Build history of the part. All positions in model axes, mm. Round coordinates to 2 decimals unless told otherwise and drop trailing zeros. Order: outer loops, then holes, each group sorted by start corner. A loop starts at its lowest first (then second) coordinate and runs counter-clockwise, first axis right, second up. Notation, with made-up numbers: (70.5, 13.5) -> (123.5, 13.5) arc R29 cw to (123.5, 43.5) -> close; hole circle Ø3 at (-18.75, -2). An arc over 180 degrees is marked (long way). Write item = value, one per line.
from build123d import *

# Parameters (mm, degrees)
SKETCH1_W           = 120
SKETCH1_H           = 120
BOSS_EXTRUDE1_DEPTH = 2
SKETCH2_R           = 1.775
CUT_EXTRUDE1_DEPTH  = 182.037166061
SKETCH3_R           = 1.775
CUT_EXTRUDE2_DEPTH  = 182.037166061
SKETCH4_W           = 3.55
SKETCH4_H           = 28
CUT_EXTRUDE3_DEPTH  = 182.037166061


with BuildPart() as part:
    # Sketch1 → Boss-Extrude1 (new body)
    with BuildSketch(Plane(origin=(0, 0, 0), x_dir=(1, 0, 0), z_dir=(0, 1, 0))):
        with Locations((104.879995502, 14.733142437)):
            Rectangle(SKETCH1_W, SKETCH1_H)
    extrude(amount=BOSS_EXTRUDE1_DEPTH)

    # Sketch2 → Cut-Extrude1 (cut, through all)
    with BuildSketch(Plane(origin=(0, 2, 0), x_dir=(1, 0, 0), z_dir=(0, 1, 0))):
        with Locations(Location((65.379995502, 30.733142437, 0), (0, 0, 270))):
            Circle(SKETCH2_R)
        with Locations(Location((65.379995502, -1.266857563, 0), (0, 0, 270))):
            Circle(SKETCH2_R)
        with Locations(Location((144.379995502, -1.266857563, 0), (0, 0, 270))):
            Circle(SKETCH2_R)
        with Locations(Location((144.379995502, 30.733142437, 0), (0, 0, 270))):
            Circle(SKETCH2_R)
    extrude(amount=-CUT_EXTRUDE1_DEPTH, mode=Mode.SUBTRACT)

    # Sketch3 → Cut-Extrude2 (cut, through all)
    with BuildSketch(Plane(origin=(0, 2, 0), x_dir=(1, 0, 0), z_dir=(0, 1, 0))):
        with Locations(Location((87.379995502, -24.766857563, 0), (0, 0, 270))):
            Circle(SKETCH3_R)
        with Locations(Location((87.379995502, 54.233142437, 0), (0, 0, 270))):
            Circle(SKETCH3_R)
        with Locations(Location((122.379995502, -24.766857563, 0), (0, 0, 270))):
            Circle(SKETCH3_R)
        with Locations(Location((122.379995502, 54.233142437, 0), (0, 0, 270))):
            Circle(SKETCH3_R)
    extrude(amount=-CUT_EXTRUDE2_DEPTH, mode=Mode.SUBTRACT)

    # Sketch4 → Cut-Extrude3 (cut, through all)
    with BuildSketch(Plane(origin=(0, 2, 0), x_dir=(1, 0, 0), z_dir=(0, 1, 0))):
        with Locations((78.879995502, 11.820412138)):
            Rectangle(SKETCH4_W, SKETCH4_H)
        with Locations((130.879995502, 11.820412138)):
            Rectangle(SKETCH4_W, SKETCH4_H)
    extrude(amount=-CUT_EXTRUDE3_DEPTH, mode=Mode.SUBTRACT)


solid = part.part
Q1. Mould opens along Z. For faces 1 (the face through (104, 0, -16)), 2 (the face through (146.14, 1.01, 1.04)), 3 (the face through (121.7, 1.014, 26.407)) say: released by +Z, released by -Z, zero draft, split by the parting line, or undercut.
Check values:
face_1 = zero draft
face_2 = undercut
face_3 = undercut
Q2. Flat gauge pin, fed straight in: pin 1 (2 mm diameter, centred on x = 87.38, z = -54.23, fed in from +Y). Where does the tip first touch, or does it go through?
Check values:
pin_1 = through
Q3. Cut at A-A, the plane y = 0.55. Give the number of separate pieces and of enclosed holes in the cut face, and give its area (3 significant figures).
Check values:
separate_pieces = 1
enclosed_holes = 10
area = 14,100 mm²
Q4. Probe probe 1 along X at (y, z) = (0.7, -5.5) (3 decimals); probe 2 along X at (y, z) = (0.4, 23.5); probe 3 along Z at (x, y) = (66.5, 0.95). List the from-to ranges inside material, lowest first.
Check values:
probe_1 = 44.88 to 77.105, 80.655 to 129.105, 132.655 to 164.88
probe_2 = 44.88 to 86.14, 88.62 to 121.14, 123.62 to 164.88
probe_3 = -74.73 to -32.11, -29.36 to -0.11, 2.64 to 45.27
Q5. Cut at B-B, the plane z = -23. List the corners of the cut face in (x, y) (3 decimals), and give its area (3 significant figures).
Check values:
outline = (44.88, 0) -> (77.105, 0) -> (77.105, 2) -> (44.88, 2) -> close; (80.655, 0) -> (129.105, 0) -> (129.105, 2) -> (80.655, 2) -> close; (132.655, 0) -> (164.88, 0) -> (164.88, 2) -> (132.655, 2) -> close
area = 226 mm²
